from build123d import *

# Parameters (mm, degrees)
BOSS_EXTRUDE1_DEPTH = 5
SKETCH2_R           = 1.5
SKETCH2_W           = 60
SKETCH2_H           = 5
CUT_EXTRUDE1_DEPTH  = 5
SKETCH4_R           = 1.5
CUT_EXTRUDE2_DEPTH  = 5


with BuildPart() as part:
    # Sketch1 → Boss-Extrude1 (new body)
    with BuildSketch(Plane.XY):
        with BuildLine():
            Line((-60, 28.75), (60, 28.75))
            ThreePointArc((60, 28.75), (67.071067812, 25.821067812), (70, 18.75))
            Line((70, 18.75), (70, -18.75))
            ThreePointArc((70, -18.75), (67.071067812, -25.821067812), (60, -28.75))
            Line((60, -28.75), (-60, -28.75))
            ThreePointArc((-60, -28.75), (-67.071067812, -25.821067812), (-70, -18.75))
            Line((-70, -18.75), (-70, 18.75))
            ThreePointArc((-70, 18.75), (-67.071067812, 25.821067812), (-60, 28.75))
        make_face()
    extrude(amount=BOSS_EXTRUDE1_DEPTH)

    # Sketch2 → Cut-Extrude1 (cut)
    with BuildSketch(Plane.XY.offset(5)):
        with Locations((60, -5.75)):
            Circle(SKETCH2_R)
        with Locations((46, -5.75)):
            Circle(SKETCH2_R)
        with Locations((46, -21.75)):
            Circle(SKETCH2_R)
        with Locations((60, -21.75)):
            Circle(SKETCH2_R)
        with Locations((-46, -5.75)):
            Circle(SKETCH2_R)
        with Locations((-46, -21.75)):
            Circle(SKETCH2_R)
        with Locations((-60, -21.75)):
            Circle(SKETCH2_R)
        with Locations((-60, -5.75)):
            Circle(SKETCH2_R)
        with Locations((0, -13.75)):
            Rectangle(SKETCH2_W, SKETCH2_H)
    extrude(amount=-CUT_EXTRUDE1_DEPTH, mode=Mode.SUBTRACT)

    # Sketch4 → Cut-Extrude2 (cut)
    with BuildSketch(Plane.XY.offset(5)):
        with Locations((7.5, 8.75)):
            Circle(SKETCH4_R)
        with Locations((-7.5, 8.75)):
            Circle(SKETCH4_R)
        with Locations((47.5, 8.75)):
            Circle(SKETCH4_R)
        with Locations((32.5, 8.75)):
            Circle(SKETCH4_R)
        with Locations((-32.5, 8.75)):
            Circle(SKETCH4_R)
        with Locations((-47.5, 8.75)):
            Circle(SKETCH4_R)
    extrude(amount=-CUT_EXTRUDE2_DEPTH, mode=Mode.SUBTRACT)


solid = part.part
Verification items for the finished model (mm, model axes). A direction names the side the tool comes from. Coordinates: 2 decimals unless noted, no trailing zeros. Loops run counter-clockwise (first coordinate to the right, second up) from the corner with the lowest first, then second, coordinate; pieces in that order, holes last. Notation, with made-up numbers: (72, -31.5) -> (130, -31.5) arc R17 cw to (130, -26.5) -> close; hole circle Ø6 at (-13, 69.25). An arc over 180 degrees is marked (long way). Answer as a JSON object with one key per item and string values. Group by question number.
Item 1: Mould release check, pull along X, two halves, no side actions. Record for faces 1 (the flat face through (0, -11.25, 3)), 2 (the cylindrical face through (67.15, -25.74, 2.46)), 3 (the flat face through (1, 0, 5)): +X half, -X half, draft (parallel to the pull), parting line (faces both ways), or undercut.
Item 2: Sectioned sample at C-C on x = -7.5. Record the boundary of the cut face in (y, z).
Item 3: Sectioned sample at A-A on y = -5.75. Record the boundary of the cut face in (x, z), plus the area to 3 significant figures.
Item 4: Sectioned sample at B-B on z = 1.55. State how many separate pieces and enclosed holes the cut face has, plus the area to 3 significant figures.
Item 5: Scan lines: probe 1 along Y at (x, z) = (-60, 3.35); probe 2 along Y at (x, z) = (24.5, 3.3); probe 3 along X at (y, z) = (-6.5, 0.4). Record each from-to range of solid material in increasing order.
Item 6: Tool access check on faces 4 (the cylindrical face through (66.99, 25.9, 2.46)), 5 (the flat face through (30, -14, 3)). Record the directions out of +Z, -Z, +X, -X, +Y, -Y that give a thin tool (end or side, any length) a straight path to the whole face; none if there is none.
Item 7: Depth check by flat-ended pin: pin 1 (2.5 mm diameter, centred on x = -32.5, y = 8.75, fed in from +Z). Enter the tip coordinate at first touch or a pass-through.
Item 8: Sectioned sample at D-D on y = 8.75. Record the boundary of the cut face in (x, z).
Evaluation:
{
 "1": {"face 1": "undercut", "face 2": "+X half", "face 3": "draft"},
 "2": {"outline": "(-28.75, 0) -> (-16.25, 0) -> (-16.25, 5) -> (-28.75, 5) -> close; (-11.25, 0) -> (7.25, 0) -> (7.25, 5) -> (-11.25, 5) -> close; (10.25, 0) -> (28.75, 0) -> (28.75, 5) -> (10.25, 5) -> close"},
 "3": {"outline": "(-70, 0) -> (-61.5, 0) -> (-61.5, 5) -> (-70, 5) -> close; (-58.5, 0) -> (-47.5, 0) -> (-47.5, 5) -> (-58.5, 5) -> close; (-44.5, 0) -> (44.5, 0) -> (44.5, 5) -> (-44.5, 5) -> close; (47.5, 0) -> (58.5, 0) -> (58.5, 5) -> (47.5, 5) -> close; (61.5, 0) -> (70, 0) -> (70, 5) -> (61.5, 5) -> close", "area": "640 mm²"},
 "4": {"separate pieces": "1", "enclosed holes": "15", "area": "7,570 mm²"},
 "5": {"probe 1": "y = -28.75 to -23.25, -20.25 to -7.25, -4.25 to 28.75", "probe 2": "y = -28.75 to -16.25, -11.25 to 28.75", "probe 3": "x = -70 to -61.3, -58.7 to -47.3, -44.7 to 44.7, 47.3 to 58.7, 61.3 to 70"},
 "6": {"face 4": "+Z, -Z, +X, +Y", "face 5": "+Z, -Z"},
 "7": {"pin 1": "passes through"},
 "8": {"outline": "(-70, 0) -> (-49, 0) -> (-49, 5) -> (-70, 5) -> close; (-46, 0) -> (-34, 0) -> (-34, 5) -> (-46, 5) -> close; (-31, 0) -> (-9, 0) -> (-9, 5) -> (-31, 5) -> close; (-6, 0) -> (6, 0) -> (6, 5) -> (-6, 5) -> close; (9, 0) -> (31, 0) -> (31, 5) -> (9, 5) -> close; (34, 0) -> (46, 0) -> (46, 5) -> (34, 5) -> close; (49, 0) -> (70, 0) -> (70, 5) -> (49, 5) -> close"}
}
